Autodesk Inventor part; units mm, degrees
ref_plane "Work Plane3" through (10.9593, -73.9067, -37.25) normal (-0.9081432, 0.4186597, 0) x (0, 0, 1)
ref_plane "Work Plane4" through (64.6996, 102.2233, -25) normal (-0.9187912, 0.3947439, 0) x (0, 0, 1)
ref_plane "Work Plane5" through (32.5419, 116.0393, -25) normal (-0.9187912, 0.3947439, 0) x (0, 0, 1)
sketch "Sketch1" plane through (0, 0, 0) normal (0, 1, 0) x (-1, 0, 0)
  line L0 (5.5, 37.25) -> (-5.5, 37.25)
  line L1 (-5.5, 37.25) -> (-5.5, -37.25)
  line L2 (-5.5, -37.25) -> (5.5, -37.25)
  line L3 (5.5, -37.25) -> (5.5, 37.25)
  line L4 (5.5, 37.25) -> (-5.5, -37.25) construction
  line L5 (-5.5, 37.25) -> (5.5, -37.25) construction
  circle A0 centre (0, 30) radius 1.5
  line L6 (5.5, 0) -> (-5.5, 0)
  circle A1 centre (0, -30) radius 1.5
  line L7 (-5.5, -25) -> (5.5, -25)
  line L8 (5.5, -25) -> (5.5, 25)
  line L9 (5.5, 25) -> (-5.5, 25)
  line L10 (-5.5, 25) -> (-5.5, -25)
  line L11 (-5.5, -25) -> (5.5, 25) construction
  line L12 (5.5, -25) -> (-5.5, 25) construction
  point P0 (0, 0)
  dimension "d0" = 11
  dimension "d1" = 74.5
  dimension "d2" = 3
  dimension "d3" = 7.25
  dimension "d28" = 50
extrude "Extrusion1" add sketch "Sketch1" along normal blind 10
sketch "Sketch2" plane through (5.5, 0, 37.25) normal (1, 0, 0) x (0, 0, -1)
  line L0 (0, 10) -> (74.5, 10)
  line L1 (0, 0) -> (74.5, 0)
  line L2 (0, 10) -> (74.5, 10)
  line L3 (74.5, 10) -> (74.5, 0)
  line L4 (74.5, 0) -> (0, 0)
  line L5 (0, 0) -> (0, 10)
  point P0 (37.25, 0)
extrude "Extrusion2" add sketch "Sketch2" along normal blind 10
sketch "Sketch3" plane through (0, 0, 0) normal (0, -1, 0) x (1, 0, 0)
  line L0 (-5.5, 37.25) -> (15.5, 37.25)
  line L1 (-5.5, -37.25) -> (15.5, -37.25)
  line L2 (15.5, 37.25) -> (4.8, 37.25)
  line L3 (4.8, 37.25) -> (4.8, -37.25)
  line L4 (4.8, -37.25) -> (15.5, -37.25)
  line L5 (15.5, -37.25) -> (15.5, 37.25)
  point P0 (0, 0)
  dimension "d9" = 10.7
extrude "Extrusion3" add sketch "Sketch3" along normal blind 76
ref_plane "Work Plane1" through (15.5, -76, -37.25) normal (-0.9081432, 0.4186597, 0) x (0, 0, 1)
ref_plane "Work Plane3" through (10.9593, -73.9067, -37.25) normal (-0.9081432, 0.4186597, 0) x (0, 0, 1)
sketch "Sketch4" plane through (10.9593, -73.9067, -37.25) normal (-0.9081432, 0.4186597, 0) x (0, 0, 1)
  circle A0 centre (37.25, 54.5) radius 2
  circle A1 centre (37.25, 54.5) radius 5.5
  circle A2 centre (27.25, 30.8) radius 2
  circle A3 centre (27.25, 30.8) radius 5.5
  line L0 (37.25, 62.5297) -> (37.25, 0)
  line L1 (0, 0) -> (74.5, 0)
  circle A4 centre (47.25, 30.8) radius 5.5
  circle A5 centre (47.25, 30.8) radius 2
  point P0 (37.25, 0)
  dimension "d13" = 4
  dimension "d14" = 11
  dimension "d15" = 4
  dimension "d16" = 11
  dimension "d19" = 10
  dimension "d20" = 23.7
  dimension "d23" = 54.5
extrude "Extrusion4" cut sketch "Sketch4" along normal blind 15 contours A0 L0 | A0 L0 A1 | L0 A0 | A0 L0 A1 | A2 | A3 | A4 | A5
extrude "Extrusion11" cut sketch "Sketch4" along normal blind 25.925 contours A0 L0 | A0 L0 A1 | L0 A0 | A0 L0 A1
extrude "Extrusion6" cut sketch "Sketch4" along normal through all contours A0 L0 | L0 A0 | A2 | A5
extrude "Extrusion7" add sketch "Sketch1" along normal blind 125 contours L3 L6 L1 L9 | L3 L7 L1 L6
sketch "Sketch5" plane through (5.5, 10, -25) normal (1, 0, 0) x (0, 0, -1)
  line L0 (0, 0) -> (0, 115)
  line L1 (0, 115) -> (0, 0)
  line L2 (0, 0) -> (-50, 0)
  line L3 (-50, 0) -> (-50, 115)
  line L4 (0, 115) -> (-50, 115)
  point P0 (-25, -10)
extrude "Extrusion8" add sketch "Sketch5" along normal blind 40
chamfer "Chamfer1" distance 40 angle 23.25 1 edges at (-5.5, 125, 0) measured on face at (-5.5, 48.3333, -8.3333)
chamfer "Chamfer2" distance 30 distance2 30 1 edges at (15.5, 10, 0)
sketch "Sketch8" plane through (11.6854, 125, -25) normal (-0.9187912, 0.3947439, 0) x (0, 0, 1)
  line L0 (0, 0) -> (0, 13.3481)
  line L1 (-12.25, -121.6327) -> (62.25, -121.6327)
  line L2 (0, 13.3481) -> (50, 13.3481)
  line L3 (50, 13.3481) -> (50, -121.6327)
  line L4 (50, -121.6327) -> (0, -121.6327)
  line L5 (0, -121.6327) -> (0, 13.3481)
  point P0 (25, -119.4616)
  point P1 (0, 0)
  dimension "d59" = 50
extrude "Extrusion12" cut sketch "Sketch8" against normal blind 22.7
ref_plane "Work Plane4" through (64.6996, 102.2233, -25) normal (-0.9187912, 0.3947439, 0) x (0, 0, 1)
ref_plane "Work Plane5" through (32.5419, 116.0393, -25) normal (-0.9187912, 0.3947439, 0) x (0, 0, 1)
ref_plane "Work Plane6" through (-5.5, 27.4944, -18.625) normal (0.3947439, 0.9187912, 0) x (0, 0, -1)
sketch "Sketch11" plane through (15.5, 10, -25) normal (0, 0, -1) x (-1, 0, 0)
  line L0 (21, 17.4944) -> (-6.8294, 82.2691)
  line L1 (21, 17.4944) -> (11, 17.4944)
  line L2 (11, 17.4944) -> (11, 13.4944)
  line L3 (11, 13.4944) -> (21, 13.4944)
  line L4 (21, 13.4944) -> (21, 17.4944)
  point P0 (15.5, -10)
  dimension "d76" = 10
  dimension "d77" = 4
extrude "Extrusion15" cut sketch "Sketch11" against normal blind 70.5
fillet "Fillet1" radius 5 2 edges at (15.5, -33, 37.25) (15.5, -33, -37.25)
sketch "Sketch12" plane through (32.5419, 116.0393, -25) normal (-0.9187912, 0.3947439, 0) x (0, 0, 1)
  line L0 (6, -0.2473) -> (44, -0.2473)
  line L1 (44, -0.2473) -> (44, -96.0989)
  line L2 (6, -96.0989) -> (6, -0.2473)
  line L3 (0, -96.3711) -> (0, 9.7527)
  line L4 (50, 9.7527) -> (50, -96.3711)
  line L5 (0, 9.7527) -> (50, 9.7527)
  line L6 (44, -96.0989) -> (44, -96.8375)
  line L7 (44, -96.8375) -> (6, -96.8375)
  line L8 (6, -96.8375) -> (6, -96.0989)
  point P0 (25, -119.4616)
  dimension "d81" = 6
  dimension "d82" = 6
  dimension "d83" = 10
extrude "Extrusion16" cut sketch "Sketch12" against normal blind 9
sketch "Sketch14" plane through (4.5, 23.4944, -25) normal (-1, 0, 0) x (0, 0, 1)
  line L0 (6, 4) -> (6, 92.3177)
  line L1 (6, 4) -> (44, 4)
  line L2 (44, 4) -> (44, 0)
  line L3 (44, 0) -> (6, 0)
  line L4 (6, 0) -> (6, 4)
  point P0 (25, -23.4944)
  point P1 (6, 19)
extrude "Extrusion18" cut sketch "Sketch14" against normal blind 7
sketch "Sketch15" plane through (15.5, 10, -25) normal (0, 0, -1) x (-1, 0, 0)
  line L0 (-30, 115) -> (-39.6875, 115)
  line L1 (-39.6875, 115) -> (-39.6875, 9.6875)
  line L2 (-30, 0) -> (-39.6875, 9.6875)
  line L3 (0, -30) -> (-30, 0)
  line L4 (21, 13.4944) -> (11, 13.4944)
  line L5 (11, 13.4944) -> (11, 17.4944)
  line L6 (11, 17.4944) -> (21, 17.4944)
  line L7 (21, 17.4944) -> (-20.8917, 115) construction
  line L8 (-20.8917, 115) -> (-30, 115)
  line L9 (-30, 0) -> (-30, 115)
  line L10 (0, -30) -> (-30, 0)
  line L11 (0, 0) -> (0, -30)
  line L12 (21, 0) -> (0, 0)
  line L13 (21, 0) -> (21, 13.4944)
  point P0 (15.5, -10)
  dimension "d91" = 135
extrude "Extrusion19" add sketch "Sketch15" against normal blind 50
sketch "Sketch16" plane through (40.811, 112.4866, -25) normal (-0.9187912, 0.3947439, 0) x (0, 0, 1)
  line L0 (6, -96.3711) -> (6, -0.2473)
  line L1 (44, -93.3357) -> (6, -93.3357)
  line L2 (6, -0.2473) -> (44, -0.2473)
  line L3 (44, -0.2473) -> (44, -93.3357)
  line L4 (44, -93.3357) -> (6, -93.3357)
  line L5 (6, -93.3357) -> (6, -0.2473)
  point P0 (25, -119.4616)
extrude "Extrusion20" cut sketch "Sketch16" against normal blind 9
properties part number "Camera Bracket"
The model under review builds one solid part; all positions refer to its coordinate system, in mm. A direction names the side the tool comes from. Coordinates: 2 decimals unless noted, no trailing zeros. Write each loop counter-clockwise with the first axis right and the second up, starting at its lowest first coordinate (ties: lowest second). Pieces come first, ordered by that corner, then holes. Notation, with made-up numbers: (5.25, 31) - (9.25, 31) arc R25 cw to (9.25, 61) - close; hole circle Ø3 at (74, 88). An arc over 180 degrees is marked (long way). Answer as a JSON object with one key per item and string values. Group by question number.
1. Add section B-B (x = 51.5). Give the boundary of the cut face in (y, z), plus the area to 3 significant figures.
2. Mouldability with a two-part tool opening along X and no side actions: class faces 6 (the face through (-5.5, 12, -1)), 7 (the face through (10.26, -39.59, -7.63)), 8 (the face through (5, 10, 31)), 9 (the face through (35.1, -0.4, -0.4)) as pulls with the +X half, pulls with the -X half, needs draft (parallel to the pull), parting line crosses it, or undercut.
3. To check wall thickness, follow probe 1 along Z at (x, y) = (0, 6); probe 2 along Y at (x, z) = (-0.5, 2.5); probe 3 along Y at (x, z) = (11.5, -29). State the ranges of each line that lie inside material, in increasing order.
4. Clearance check with flat-ended pins moving along their axes: pin 1 Ø3 at (x, z) = (-1, -21) entering from -Y; pin 2 Ø1.8 at (x, z) = (0, -30) entering from +Y; pin 3 Ø6 at (x, y) = (29, 15.5) entering from +Z; pin 4 Ø5 at (x, z) = (28.5, -23) entering from -Y. State where each tip first meets the part, or that it passes through.
5. Add section A-A (x = 43.5). Give the boundary of the cut face in (y, z).
6. Machinability: for faces 1 (the face through (5, 10, -31)), 2 (the face through (4.8, -37, 1)), 3 (the face through (-1, 27.494, -22)), 4 (the face through (10.263, -13.488, 2.367)), 5 (the face through (20, 70, 19)), which of the approach directions +Z, -Z, +X, -X, +Y, -Y give a long, thin tool a straight path to every point of the face, cutting with its end or side? Answer none if there is none.
Findings:
{
 "1": {"outline": "(16, -25) - (125, -25) - (125, 25) - (16, 25) - close", "area": "5,450 mm²"},
 "2": {"face 6": "pulls with the -X half", "face 7": "undercut", "face 8": "needs draft", "face 9": "pulls with the +X half"},
 "3": {"probe 1": "-37.25 to -31.5, -28.5 to 28.5, 31.5 to 37.25", "probe 2": "0 to 23.49", "probe 3": "-76 to 10"},
 "4": {"pin 1": "y = 0", "pin 2": "through", "pin 3": "z = 25", "pin 4": "y = -9.5"},
 "5": {"outline": "(8, -25) - (125, -25) - (125, 25) - (8, 25) - close; hole (95.94, -19) - (111.06, -19) - (111.06, 19) - (95.94, 19) - close"},
 "6": {"face 1": "-Z, +X, -X, +Y", "face 2": "+Z, -Z, -X, -Y", "face 3": "+Z, -Z, -X", "face 4": "none", "face 5": "-X"}
}
